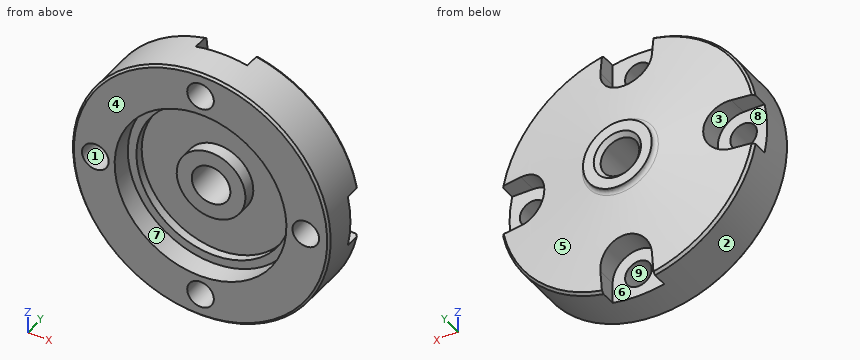
from build123d import *

# Parameters (mm, degrees)
SKETCH_1_R               = 15
EXTRUDE_314_DEPTH        = 8
SKETCH_3_R               = 10
CUT_EXTRUDE_1_DEPTH      = 2.5
SKETCH_5_R               = 9
CUT_EXTRUDE_3_DEPTH      = 1
SKETCH_6_R               = 4
EXTRUDE_2_DEPTH          = 1.5
SKETCH_7_R               = 2.25
CUT_EXTRUDE_4_DEPTH      = 23.671568098
CHAMFER_3_SIZE           = 0.5
CHAMFER_4_SIZE           = 0.25
CHAMFER_4_SIZE_2         = 0.292152675
CHAMFER_5_SIZE           = 0.25
FILLET_1_R               = 0.5
CUT_EXTRUDE_START        = 4
CUT_EXTRUDE_6_DEPTH      = 19.671568133
SKETCH_9_R               = 1.55
CUT_EXTRUDE_7_DEPTH      = 22.587033163
PATTERN_CIRCULAR_1_COUNT = 4


with BuildPart() as part:
    # Sketch 1 → Extrude 314 (new body)
    with BuildSketch(Plane(origin=(0, 0, 0), x_dir=(1, 0, 0), z_dir=(0, 1, 0))):
        with Locations(Location((0, 0, 0), (0, 0, 270))):
            Circle(SKETCH_1_R)
    extrude(amount=EXTRUDE_314_DEPTH)

    # Sketch 2 → Cut-Revolve 1 (revolve, cut)
    with BuildSketch(Plane.XY, mode=Mode.PRIVATE) as cut_revolve_1_sk:
        Polygon((4, 8), (15, 8), (15, 6), (4, 7.5), align=None)
    revolve(cut_revolve_1_sk.sketch.rotate(Axis((0, -1.597938144, 0), (0, 1, 0)), 90), axis=Axis((0, -1.597938144, 0), (0, 1, 0)), mode=Mode.SUBTRACT)

    # Sketch 3 → Cut-Extrude 1 (cut)
    with BuildSketch(Plane(origin=(0, 0, 0), x_dir=(-1, 0, 0), z_dir=(0, -1, 0))):
        with Locations(Location((0, 0, 0), (0, 0, 90))):
            Circle(SKETCH_3_R)
    extrude(amount=-CUT_EXTRUDE_1_DEPTH, mode=Mode.SUBTRACT)

    # Sketch 5 → Cut-Extrude 3 (cut)
    with BuildSketch(Plane.XZ.offset(-2.5)):
        with Locations(Location((0, 0, 0), (0, 0, 270))):
            Circle(SKETCH_5_R)
    extrude(amount=-CUT_EXTRUDE_3_DEPTH, mode=Mode.SUBTRACT)

    # Sketch 6 → Extrude 2 (add)
    with BuildSketch(Plane.XZ.offset(-3.5)):
        with Locations(Location((0, 0, 0), (0, 0, 270))):
            Circle(SKETCH_6_R)
    extrude(amount=EXTRUDE_2_DEPTH)

    # Sketch 7 → Cut-Extrude 4 (cut, through all)
    with BuildSketch(Plane(origin=(0, 8, 0), x_dir=(1, 0, 0), z_dir=(0, 1, 0))):
        with Locations(Location((0, 0, 0), (0, 0, 270))):
            Circle(SKETCH_7_R)
    extrude(amount=-CUT_EXTRUDE_4_DEPTH, mode=Mode.SUBTRACT)

    # Chamfer 3
    chamfer_3_edges = [part.edges().sort_by_distance(p)[0] for p in [
        (0, 8, -2.25),
    ]]
    chamfer(chamfer_3_edges, length=CHAMFER_3_SIZE)

    # Chamfer 4
    # the kernel refuses this chamfer: 0.292152675, 0.25 mm, written as the material it takes off along each edge
    with BuildSketch(Plane(origin=(0, 6, 0), x_dir=(0, 0, 1), z_dir=(-1, 0, 0))) as chamfer_4_piece_1:
        Polygon((15 - CHAMFER_4_SIZE * 0.990830168044, CHAMFER_4_SIZE * 0.135113204733), (15, -CHAMFER_4_SIZE_2), (15, 0), align=None)
    revolve(axis=Axis((0, 6, 0), (0, 1, 0)), revolution_arc=180, mode=Mode.SUBTRACT)
    with BuildSketch(Plane(origin=(0, 6, 0), x_dir=(0, 0, -1), z_dir=(1, 0, 0))) as chamfer_4_piece_2:
        Polygon((15 - CHAMFER_4_SIZE * 0.990830168044, CHAMFER_4_SIZE * 0.135113204733), (15, -CHAMFER_4_SIZE_2), (15, 0), align=None)
    revolve(axis=Axis((0, 6, 0), (0, 1, 0)), revolution_arc=180, mode=Mode.SUBTRACT)

    # Chamfer 5
    chamfer_5_edges = [part.edges().sort_by_distance(p)[0] for p in [
        (0, 0, -15),
    ]]
    chamfer(chamfer_5_edges, length=CHAMFER_5_SIZE)

    # Fillet 1
    fillet_1_edges = [part.edges().sort_by_distance(p)[0] for p in [
        (0, 7.5, 4),
    ]]
    fillet(fillet_1_edges, radius=FILLET_1_R)

    # Sketch 8 → Cut-Extrude 6 (cut, through all)
    with BuildSketch(Plane(origin=(0, 0, 0), x_dir=(1, 0, 0), z_dir=(0, 1, 0)).offset(CUT_EXTRUDE_START)):
        with BuildLine():
            Line((3, 12.25), (3, 14.696938457))
            ThreePointArc((3, 14.696938457), (0, 15), (-3, 14.696938457))
            Line((-3, 14.696938457), (-3, 12.25))
            ThreePointArc((-3, 12.25), (0, 9.25), (3, 12.25))
        make_face()
    cut_extrude_6 = extrude(amount=CUT_EXTRUDE_6_DEPTH, mode=Mode.SUBTRACT)

    # Sketch 9 → Cut-Extrude 7 (cut, through all)
    with BuildSketch(Plane(origin=(0, 4, 0), x_dir=(1, 0, 0), z_dir=(0, 1, 0))):
        with Locations(Location((0, 12.25, 0), (0, 0, 270))):
            Circle(SKETCH_9_R)
    cut_extrude_7 = extrude(amount=-CUT_EXTRUDE_7_DEPTH, mode=Mode.SUBTRACT)

    # Pattern Circular 1: Cut-Extrude 6, Cut-Extrude 7 ×4 about axis
    pattern_circular_1_axis = Axis((0, 0, 0), (0, 1, 0))
    add([cut_extrude_6.rotate(pattern_circular_1_axis, i * 360 / PATTERN_CIRCULAR_1_COUNT) for i in range(1, PATTERN_CIRCULAR_1_COUNT)], mode=Mode.SUBTRACT)
    add([cut_extrude_7.rotate(pattern_circular_1_axis, i * 360 / PATTERN_CIRCULAR_1_COUNT) for i in range(1, PATTERN_CIRCULAR_1_COUNT)], mode=Mode.SUBTRACT)


solid = part.part
The model under review builds one solid part; all positions refer to its coordinate system, in mm. Face numbers are marked on the shaded views. A direction names the side the tool comes from. Coordinates: 2 decimals unless noted, no trailing zeros. Answer in a Markdown table with one row per item.
(1) Machinability: for the marked faces 5, 6, 7, 8 and 9, which of the approach directions +Z, -Z, +X, -X, +Y, -Y give a long, thin tool a straight path to every point of the face, cutting with its end or side? Answer none if there is none.
Answers:
| item | result |
|---|---|
| face 5 | +Y |
| face 6 | -Z, +Y |
| face 7 | -Y |
| face 8 | -X, +Y |
| face 9 | +Y, -Y |
(2) The part is to be moulded in two halves that separate along X. For the marked faces 1, 2, 3 and 4, say which applies: +X half, -X half, draft (parallel to the pull), parting line (faces both ways), or undercut.
Answers:
| item | result |
|---|---|
| face 1 | undercut |
| face 2 | parting line |
| face 3 | -X half |
| face 4 | draft |
(3) Wall thickness on line 1 along X through (y, z) = (3, -3.5); line 2 along X through (y, z) = (2.25, 2.5); line 3 along X through (y, z) = (2.25, 8.5): over which ranges is each line inside the solid? List them lowest first.
Answers:
| item | result |
|---|---|
| line 1 | -14.59 to -8.29, -1.94 to 1.94, 8.29 to 14.59 |
| line 2 | -14.79 to -9.68, -3.12 to 3.12, 9.68 to 14.79 |
| line 3 | -12.36 to -5.27, 5.27 to 12.36 |
(4) Consider section A-A (z = 0). State how many separate pieces and enclosed holes the cut face has, plus the area to 3 significant figures.
Answers:
| item | result |
|---|---|
| separate pieces | 4 |
| enclosed holes | 0 |
| area | 77.0 mm² |
(5) Insertion check: pin 1 (8 mm diameter, centred on x = 6.5, z = -11, fed in from -Y); pin 2 (1.5 mm diameter, centred on x = 8.5, y = 3.5, fed in from +Z); pin 3 (1.7 mm diameter, centred on x = 13, z = 0, fed in from +Y); pin 4 (1.2 mm diameter, centred on x = -14, y = 5.5, fed in from +Z). Each pin has a flat end and moves straight along its axis. Give the tip position at first contact, or say it passes through.
Answers:
| item | result |
|---|---|
| pin 1 | y = 0 |
| pin 2 | z = 12.84 |
| pin 3 | y = 4 |
| pin 4 | z = 6.74 |
